Check sheet for the modelled part. Datum: model origin and axes. Units: mm. Face numbers are marked on the shaded views. A direction names the side the tool comes from. Round coordinates to 2 decimals unless told otherwise and drop trailing zeros. Order: outer loops, then holes, each group sorted by start corner. A loop starts at its lowest first (then second) coordinate and runs counter-clockwise, first axis right, second up.
(1) Sectioned sample at A-A, the plane x = 0. Enter the section's corners in (y, z).
(2) Depth check by flat-ended pin: pin 1 (0.6 mm diameter, centred on y = 0, z = -1, fed in from -X); pin 2 (1.5 mm diameter, centred on x = 1, z = 22, fed in from +Y); pin 3 (1.5 mm diameter, centred on y = -0.5, z = 8.5, fed in from -X). Enter the tip coordinate at first touch or a pass-through.
(3) Sectioned sample at C-C, the plane z = 6. Enter the section's corners in (x, y), and give its area (3 significant figures).
(4) Thickness scan on probe 1 along Y at (x, z) = (0.55, 4.5); probe 2 along Z at (x, y) = (-0.85, 1.7); probe 3 along Z at (x, y) = (0.6, -0.35). Record the ranges inside material, lowest first.
(5) Tool access check on the marked faces 1 and 2. Record the directions out of +Z, -Z, +X, -X, +Y, -Y that give a thin tool (end or side, any length) a straight path to the whole face; none if there is none.
Autodesk Inventor part; units mm, degrees
ref_plane "YZ Plane" through (0, 0, 0) normal (1, 0, 0) x (0, 1, 0)
ref_plane "XZ Plane" through (0, 0, 0) normal (0, 1, 0) x (-1, 0, 0)
ref_plane "XY Plane" through (0, 0, 0) normal (0, 0, 1) x (1, 0, 0)
sketch "Sketch1" plane through (0, 0, 0) normal (0, 0, 1) x (1, 0, 0)
  circle A0 centre (0, 0) radius 1.5
  dimension "d0" = 3
extrude "Extrusion1" add sketch "Sketch1" along normal blind 30
fillet "Fillet1" radius 0.1 1 edges at (-1.5, 0, 30)
sketch "Sketch2" plane through (0, 0, 0) normal (0, 0, -1) x (-1, 0, 0)
  circle A0 centre (0, 0) radius 2.5
  dimension "d4" = 5
extrude "Extrusion2" add sketch "Sketch2" along normal blind 1
sketch "Sketch3" plane through (0, 0, -1) normal (0, 0, -1) x (-1, 0, 0)
  line L0 (-1.4142, 0.5) -> (1.4142, 0.5)
  line L1 (1.4142, 0.5) -> (1.4142, -0.5)
  line L2 (1.4142, -0.5) -> (-1.4142, -0.5)
  line L3 (-1.4142, -0.5) -> (-1.4142, 0.5)
  line L4 (-1.4142, 0.5) -> (1.4142, -0.5) construction
  line L5 (1.4142, 0.5) -> (-1.4142, -0.5) construction
  line L6 (0.5, 1.4142) -> (-0.5, 1.4142)
  line L7 (-0.5, 1.4142) -> (-0.5, -1.4142)
  line L8 (-0.5, -1.4142) -> (0.5, -1.4142)
  line L9 (0.5, -1.4142) -> (0.5, 1.4142)
  line L10 (0.5, 1.4142) -> (-0.5, -1.4142) construction
  line L11 (-0.5, 1.4142) -> (0.5, -1.4142) construction
  point P0 (0, 0)
  point P1 (0, 0)
  point P2 (0, 0)
  dimension "d8" = 1
  dimension "d9" = 1
extrude "Extrusion3" cut sketch "Sketch3" against normal blind 0.5
fillet "Fillet2" radius 0.6 1 edges at (2.5, 0, -1)
properties part number "M3-2"
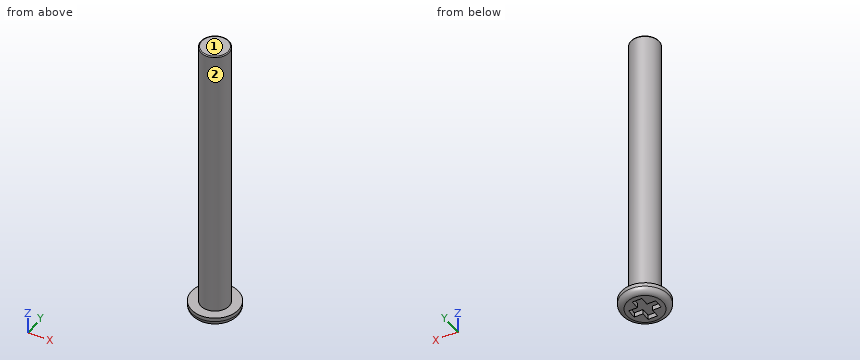
Derived:
1. outline: (-2.5, -0.4) arc R0.6 ccw to (-1.9, -1) - (-1.41, -1) - (-1.41, -0.5) - (1.41, -0.5) - (1.41, -1) - (1.9, -1) arc R0.6 ccw to (2.5, -0.4) - (2.5, 0) - (1.5, 0) - (1.5, 29.9) arc R0.1 ccw to (1.4, 30) - (-1.4, 30) arc R0.1 ccw to (-1.5, 29.9) - (-1.5, 0) - (-2.5, 0) - close
2. pin 1: stops at x = -2.42
2. pin 2: stops at y = 1.48
2. pin 3: stops at x = -1.5
3. outline: circle Ø3 at (0, 0)
3. area: 7.07 mm2
4. probe 1: y = -1.4 to 1.4
4. probe 2: z = -1 to 0
4. probe 3: z = -0.5 to 30
5. face 1: +Z, +X, -X, +Y, -Y
5. face 2: +Z
